Input: part model. Units: mm. Frame: model coordinates. Round coordinates to 2 decimals unless told otherwise and drop trailing zeros. Loops run counter-clockwise (first coordinate to the right, second up) from the corner with the lowest first, then second, coordinate; pieces in that order, holes last. Notation, with made-up numbers: M 1,-24.5 L 14,-24.5 A28 cw 14,-4.5 Z; hole C 34.5,82.25 d1. An arc over 180 degrees is marked long. Use one line per item in the form item = value. Start each with the question number.
Q1. First-contact query: P1, Ø10, axis at x = -8, z = -250.5, coming from the -Y side (3 decimals). Flat tip, straight axial feed; report the tip coordinate or a pass-through.
Q2. Ray query, line 1 along X through (y, z) = (-0.15, -801.5); line 2 along Y through (x, z) = (-18.75, -845.5) (3 decimals); line 3 along X through (y, z) = (-2.1, -339). Return the intervals inside material, ascending.
Q3. Section query A-A, the plane z = -155. Output: boundary loops of the cut face in (x, y) (3 decimals).
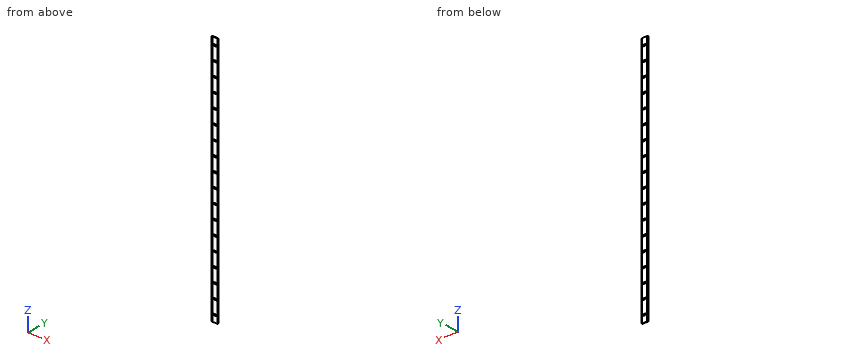
```python
from build123d import *

# Parameters (mm, degrees)
BOSS_EXTRUDE1_DEPTH = 900
FILLET1_R           = 0.2
CUT_EXTRUDE1_DEPTH  = 2.375
LPATTERN1_COUNT     = 18
LPATTERN1_PITCH     = 50


with BuildPart() as part:
    # Sketch1 → Boss-Extrude1 (new body)
    with BuildSketch(Plane.XY):
        Polygon((0, 0), (-19.2062, 0), (-19.5291, 0), (-21.9041, -2.375), (-19.5291, -4.75), (-19.2062, -4.75), (-19.2062, -2.375), (0, -2.375), align=None)
    extrude(amount=-BOSS_EXTRUDE1_DEPTH)

    # Fillet1
    fillet1_edges = [part.edges().sort_by_distance(p)[0] for p in [
        (0, -2.375, -450),
        (-19.2062, -4.75, -450),
        (-19.5291, -4.75, -450),
        (-21.9041, -2.375, -450),
        (-19.5291, 0, -450),
        (0, 0, -450),
    ]]
    fillet(fillet1_edges, radius=FILLET1_R)

    # Sketch2 → Cut-Extrude1 (cut)
    with BuildSketch(Plane(origin=(0, 0, 0), x_dir=(1, 0, 0), z_dir=(0, 1, 0))):
        with BuildLine():
            Line((-12.823128644, 27.625), (-6.823128644, 27.625))
            ThreePointArc((-6.823128644, 27.625), (-4.198128644, 25), (-6.823128644, 22.375))
            Line((-6.823128644, 22.375), (-12.823128644, 22.375))
            ThreePointArc((-12.823128644, 22.375), (-15.448128644, 25), (-12.823128644, 27.625))
        make_face()
    cut_extrude1 = extrude(amount=-CUT_EXTRUDE1_DEPTH, mode=Mode.SUBTRACT)

    # LPattern1: Cut-Extrude1 ×18
    with Locations(*[(0, 0, -i * LPATTERN1_PITCH) for i in range(1, LPATTERN1_COUNT)]):
        add(cut_extrude1, mode=Mode.SUBTRACT)


solid = part.part
```
Results found:
q1.P1 = -2.375
q2.line_1 = -19.68 to -0.01
q2.line_2 = -2.375 to 0
q2.line_3 = -21.63 to 0
q3.outline = M -21.763,-2.516 L -19.588,-4.691 A0.2 ccw -19.446,-4.75 L -19.406,-4.75 A0.2 ccw -19.206,-4.55 L -19.206,-2.375 L -0.2,-2.375 A0.2 ccw 0,-2.175 L 0,-0.2 A0.2 ccw -0.2,0 L -19.446,0 A0.2 ccw -19.588,-0.059 L -21.763,-2.234 A0.2 ccw Z
